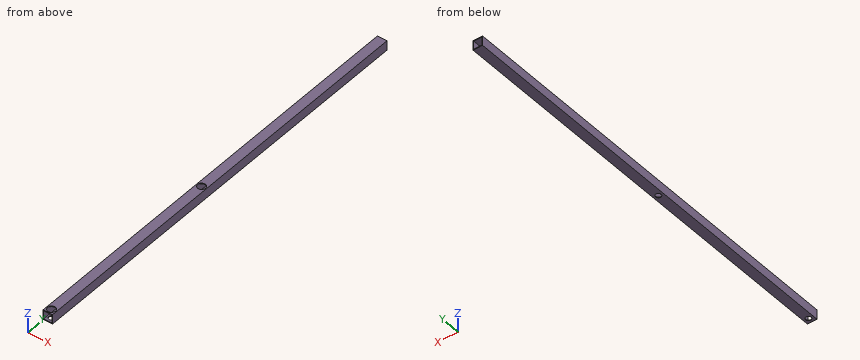
```python
from build123d import *

# Parameters (mm, degrees)
SKETCH1_W           = 44.45
SKETCH1_H           = 44.45
SKETCH1_W_2         = 38.1
SKETCH1_H_2         = 38.1
BOSS_EXTRUDE1_DEPTH = 1981.2
CUT_EXTRUDE1_REACH  = 46.45
SKETCH2_R           = 18.25625
CUT_EXTRUDE2_REACH  = 46.45
SKETCH4_R           = 12.7


with BuildPart() as part:
    # Sketch1 → Boss-Extrude1 (new body)
    with BuildSketch(Plane(origin=(0, 0, 0), x_dir=(1, 0, 0), z_dir=(0, 1, 0))):
        with Locations((22.225, 22.225)):
            Rectangle(SKETCH1_W, SKETCH1_H)
        with Locations((22.225, 22.225)):
            Rectangle(SKETCH1_W_2, SKETCH1_H_2, mode=Mode.SUBTRACT)
    extrude(amount=BOSS_EXTRUDE1_DEPTH)

    # Sketch2 → Cut-Extrude1 (cut, up to next)
    with BuildSketch(Plane.XY, mode=Mode.PRIVATE) as cut_extrude1_sk1:
        with Locations((22.225, 22.225)):
            Circle(SKETCH2_R)
    cut_extrude1_tool1 = extrude(cut_extrude1_sk1.sketch, amount=-CUT_EXTRUDE1_REACH, mode=Mode.PRIVATE) & part.part
    add(cut_extrude1_tool1.solids().sort_by_distance((22.225, 22.225, 0))[0], mode=Mode.SUBTRACT)
    # Sketch2 → Cut-Extrude1 (cut, up to next)
    with BuildSketch(Plane.XY, mode=Mode.PRIVATE) as cut_extrude1_sk2:
        with Locations((22.225, 911.225)):
            Circle(SKETCH2_R)
    cut_extrude1_tool2 = extrude(cut_extrude1_sk2.sketch, amount=-CUT_EXTRUDE1_REACH, mode=Mode.PRIVATE) & part.part
    add(cut_extrude1_tool2.solids().sort_by_distance((22.225, 911.225, 0))[0], mode=Mode.SUBTRACT)

    # Sketch4 → Cut-Extrude2 (cut, up to next)
    with BuildSketch(Plane(origin=(0, 0, -44.45), x_dir=(-1, 0, 0), z_dir=(0, 0, -1)), mode=Mode.PRIVATE) as cut_extrude2_sk1:
        with Locations((-22.225, 911.225)):
            Circle(SKETCH4_R)
    cut_extrude2_tool1 = extrude(cut_extrude2_sk1.sketch, amount=-CUT_EXTRUDE2_REACH, mode=Mode.PRIVATE) & part.part
    add(cut_extrude2_tool1.solids().sort_by_distance((22.225, 911.225, -44.45))[0], mode=Mode.SUBTRACT)
    # Sketch4 → Cut-Extrude2 (cut, up to next)
    with BuildSketch(Plane(origin=(0, 0, -44.45), x_dir=(-1, 0, 0), z_dir=(0, 0, -1)), mode=Mode.PRIVATE) as cut_extrude2_sk2:
        with Locations((-22.225, 22.225)):
            Circle(SKETCH4_R)
    cut_extrude2_tool2 = extrude(cut_extrude2_sk2.sketch, amount=-CUT_EXTRUDE2_REACH, mode=Mode.PRIVATE) & part.part
    add(cut_extrude2_tool2.solids().sort_by_distance((22.225, 22.225, -44.45))[0], mode=Mode.SUBTRACT)


solid = part.part
```
Geometry check sheet. Reference: the model listing, model coordinates, mm. Round coordinates to 2 decimals unless told otherwise and drop trailing zeros. Loops run counter-clockwise (first coordinate to the right, second up) from the corner with the lowest first, then second, coordinate; pieces in that order, holes last. Notation, with made-up numbers: (39.25, 57.5) - (60.25, 57.5) arc R9 ccw to (60.25, 67.5) - close; hole circle Ø5 at (74, -27). An arc over 180 degrees is marked (long way). Write each question's results on one line, items separated by ' | '. Start each with the question number.
Q1. Cross-section at B-B on y = 315.5. Enter the section's corners in (x, z) (3 decimals).
Q2. Cross-section at A-A on z = -19.5. Enter the section's corners in (x, y) (3 decimals), and give its area (3 significant figures).
Q3. Cross-section at C-C on x = 18. Enter the section's corners in (y, z) (3 decimals).
Q4. Thickness scan on line 1 (X direction, y = 1412, z = -37) (3 decimals); line 2 (Z direction, x = 33, y = 933) (3 decimals); line 3 (Y direction, x = 29.5, z = -42). Record the ranges inside material, lowest first. Write a range as [from, to].
Answers below:
1) outline: (0, -44.45) - (44.45, -44.45) - (44.45, 0) - (0, 0) - close; hole (3.175, -41.275) - (41.275, -41.275) - (41.275, -3.175) - (3.175, -3.175) - close
2) outline: (0, 0) - (3.175, 0) - (3.175, 1981.2) - (0, 1981.2) - close; (41.275, 0) - (44.45, 0) - (44.45, 1981.2) - (41.275, 1981.2) - close | area: 12,600 mm²
3) outline: (0, -44.45) - (10.248, -44.45) - (10.248, -41.275) - (0, -41.275) - close; (0, -3.175) - (4.464, -3.175) - (4.464, 0) - (0, 0) - close; (34.202, -44.45) - (899.248, -44.45) - (899.248, -41.275) - (34.202, -41.275) - close; (39.986, -3.175) - (893.464, -3.175) - (893.464, 0) - (39.986, 0) - close; (923.202, -44.45) - (1981.2, -44.45) - (1981.2, -41.275) - (923.202, -41.275) - close; (928.986, -3.175) - (1981.2, -3.175) - (1981.2, 0) - (928.986, 0) - close
4) line 1: x = [0, 3.175], [41.275, 44.45] | line 2: z = [-44.45, -41.275], [-3.175, 0] | line 3: y = [0, 11.82], [32.63, 900.82], [921.63, 1981.2]
